from build123d import *

# Parameters (mm, degrees)
SKETCH2_W          = 177.8
SKETCH2_H          = 38.1
CUT_EXTRUDE1_DEPTH = 25.4
CHAMFER1_SIZE      = 12.7
CHAMFER2_SIZE      = 25.4


with BuildPart() as part:
    # Sketch1 → Revolve1 (revolve)
    with BuildSketch(Plane.XY, mode=Mode.PRIVATE) as revolve1_sk:
        Polygon((0, 0), (0, 101.6), (63.5, 101.6), (63.5, 50.8), (25.4, 50.8), (25.4, 0), align=None)
    revolve(revolve1_sk.sketch.rotate(Axis((0, 0, 0), (0, 1, 0)), 90), axis=Axis((0, 0, 0), (0, 1, 0)))

    # Sketch2 → Cut-Extrude1 (cut)
    with BuildSketch(Plane(origin=(0, 101.6, 0), x_dir=(1, 0, 0), z_dir=(0, 1, 0))):
        Rectangle(SKETCH2_W, SKETCH2_H)
    extrude(amount=-CUT_EXTRUDE1_DEPTH, mode=Mode.SUBTRACT)

    # Chamfer1
    chamfer1_edges = [part.edges().sort_by_distance(p)[0] for p in [
        (0, 101.6, 19.05),
        (0, 101.6, -19.05),
    ]]
    chamfer(chamfer1_edges, length=CHAMFER1_SIZE)

    # Chamfer2
    chamfer2_edges = [part.edges().sort_by_distance(p)[0] for p in [
        (0, 50.8, 63.5),
    ]]
    chamfer(chamfer2_edges, length=CHAMFER2_SIZE - 0.0001)  # a hair under: the kernel refuses the full size


solid = part.part
Can you work these out from the model? Positions are in its coordinate system, mm. A direction names the side the tool comes from. Coordinates: 2 decimals unless noted, no trailing zeros. Write each loop counter-clockwise with the first axis right and the second up, starting at its lowest first coordinate (ties: lowest second). Pieces come first, ordered by that corner, then holes. Notation, with made-up numbers: (35, -21.5) - (74, -21.5) arc R29 ccw to (74, 11.5) - close; hole circle Ø2 at (11, 64). An arc over 180 degrees is marked (long way). Return JSON: item names as keys, results as strings. Group by question number.
Item 1: If we section it at C-C (x = 0): Write out the boundary of the cut face in (y, z), then the cut area to 3 significant figures.
Item 2: I'm going to push flat-ended pins straight in: pin 1 Ø1.5 at (x, z) = (6.5, -13.5) entering from +Y; pin 2 Ø10 at (x, y) = (0.5, 60.5) entering from -Z; pin 3 Ø3 at (x, y) = (-24.5, 69) entering from +Z. Where does each tip first touch, or does it pass through?
Item 3: If we section it at D-D (y = 26.5): Write out the boundary of the cut face in (x, z), then the cut area to 3 significant figures.
Item 4: Which directions (+Z, -Z, +X, -X, +Y, -Y) give clear straight access to the entire face, cutting with the end or side of a thin tool? Please do faces 5 (the face through (15.456, 25.044, 20.157)), 6 (the face through (-19.07, 88.72, -60.57)), 7 (the face through (-0.85, 95.34, 25.49)).
Item 5: Please list where these lines run through material, in increasing order: probe 1 along Y at (x, z) = (-26, -15.5); probe 2 along Z at (x, y) = (-11.5, 87.5); probe 3 along Y at (x, z) = (35, 19).
Item 6: If we section it at B-B (y = 78.5): Write out the boundary of the cut face in (x, z), then the cut area to 3 significant figures.
Item 7: We'd pull the mould along Z, two halves only. Please class faces 1 (the face through (-1.729, 52.033, 39.295)), 2 (the face through (-1, 76.2, 0)), 3 (the face through (-1, 101.6, -44)), 4 (the face through (-1, 83, 19.05)): pulls with the +Z half, pulls with the -Z half, needs draft (parallel to the pull), parting line crosses it, or undercut.
Return value:
{
 "1": {"outline": "(0, -25.4) - (50.8, -25.4) - (50.8, -38.1) - (76.2, -63.5) - (101.6, -63.5) - (101.6, -31.75) - (88.9, -19.05) - (76.2, -19.05) - (76.2, 19.05) - (88.9, 19.05) - (101.6, 31.75) - (101.6, 63.5) - (76.2, 63.5) - (50.8, 38.1) - (50.8, 25.4) - (0, 25.4) - close", "area": "7,260 mm^2"},
 "2": {"pin 1": "stops at y = 76.2", "pin 2": "stops at z = -52.8", "pin 3": "stops at z = 52.49"},
 "3": {"outline": "circle Ø50.8 at (0, 0)", "area": "2,030 mm^2"},
 "4": {"face 5": "-Y", "face 6": "+Y, -Y", "face 7": "+X, -X, +Y"},
 "5": {"probe 1": "y = 50.8 to 76.2", "probe 2": "z = -62.45 to -19.05, 19.05 to 62.45", "probe 3": "y = 52.52 to 76.2"},
 "6": {"outline": "(-60.58, -19.05) arc R63.5 ccw to (60.58, -19.05) - close; (-60.58, 19.05) - (60.58, 19.05) arc R63.5 ccw to start", "area": "7,900 mm^2"},
 "7": {"face 1": "parting line crosses it", "face 2": "undercut", "face 3": "needs draft", "face 4": "undercut"}
}
